from build123d import *

# Parameters (mm, degrees)
SKETCH_1_R               = 1.1
EXTRUDE_2_DEPTH          = 4.5
FILLET_1_R               = 7
FILLET_2_R               = 14
FILLET_3_R               = 2
CUT_EXTRUDE_1_DEPTH      = 33.524221985
CUT_EXTRUDE_1_DEPTH_BACK = 33.524221985


with BuildPart() as part:
    # 草图1 → 凸台-拉伸2 (new body)
    with BuildSketch(Plane.XY):
        with BuildLine():
            Line((6.017486991, 19.788810031), (-7.057549395, 16.285364591))
            Line((-7.057549395, 16.285364591), (-7.057549395, -16.139577348))
            Line((-7.057549395, -16.139577348), (-7.057549395, -28.167744528))
            Line((-7.057549395, -28.167744528), (6.017486991, -31.671189969))
            Line((6.017486991, -31.671189969), (7.089384541, -30.477023749))
            ThreePointArc((7.089384541, -30.477023749), (3.917486991, -28.671189969), (7.089384541, -26.865356188))
            Line((7.089384541, -26.865356188), (6.017486991, -25.671189969))
            Line((6.017486991, -25.671189969), (-2.887475269, -24.892106722))
            Line((-2.887475269, -24.892106722), (-2.887475269, 13.009726784))
            Line((-2.887475269, 13.009726784), (6.017486991, 13.788810031))
            Line((6.017486991, 13.788810031), (7.089384541, 14.982976251))
            ThreePointArc((7.089384541, 14.982976251), (3.917486991, 16.788810031), (7.089384541, 18.594643812))
            Line((7.089384541, 18.594643812), (6.017486991, 19.788810031))
        make_face()
        with Locations((-4.879152463, 4.788810031)):
            Circle(SKETCH_1_R, mode=Mode.SUBTRACT)
        with Locations((-4.879152463, -16.671189969)):
            Circle(SKETCH_1_R, mode=Mode.SUBTRACT)
    extrude(amount=EXTRUDE_2_DEPTH)

    # 圆角1
    fillet_1_edges = [part.edges().sort_by_distance(p)[0] for p in [
        (-2.887475269, 13.009726784, 2.25),
        (-2.887475269, -24.892106722, 2.25),
    ]]
    fillet(fillet_1_edges, radius=FILLET_1_R)

    # 圆角2
    fillet_2_edges = [part.edges().sort_by_distance(p)[0] for p in [
        (-7.057549395, -28.167744528, 2.25),
        (-7.057549395, 16.285364591, 2.25),
    ]]
    fillet(fillet_2_edges, radius=FILLET_2_R)

    # 圆角3
    fillet_3_edges = [part.edges().sort_by_distance(p)[0] for p in [
        (6.017486991, 13.788810031, 2.25),
        (6.017486991, -25.671189969, 2.25),
        (6.017486991, -31.671189969, 2.25),
        (6.017486991, 19.788810031, 2.25),
    ]]
    fillet(fillet_3_edges, radius=FILLET_3_R)

    # 草图2 → 切除-拉伸1 (cut, two sides: drawn at the far end of the back side and taken through both)
    with BuildSketch(Plane(origin=(0, 0, 0), x_dir=(1, 0, 0), z_dir=(0, 1, 0)).offset(-CUT_EXTRUDE_1_DEPTH_BACK)):
        Polygon((-9.937735325, -0.89235354), (-9.653427695, 2.8886559), (6.091848462, 2.8886559), (7.089384541, 0), (-4.928773799, -0.62984499), (-9.504604651, -0.62984499), align=None)
        Polygon((7.089384541, -4.5), (-9.927872999, -3.608163323), (-9.667318366, -5.613598375), (7.089384541, -5.407507841), align=None)
    extrude(amount=CUT_EXTRUDE_1_DEPTH + CUT_EXTRUDE_1_DEPTH_BACK, mode=Mode.SUBTRACT)


solid = part.part
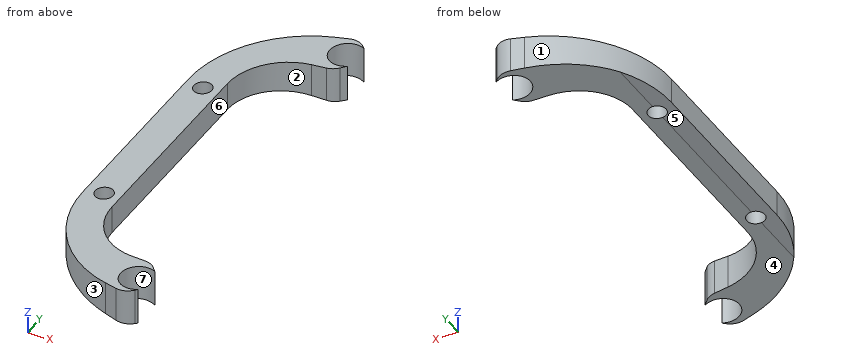
Model file for the job. Use its own axes, mm. Face numbers are marked on the shaded views. A direction names the side the tool comes from. Round coordinates to 2 decimals unless told otherwise and drop trailing zeros. Order: outer loops, then holes, each group sorted by start corner. A loop starts at its lowest first (then second) coordinate and runs counter-clockwise, first axis right, second up. Notation, with made-up numbers: M 25,56.5 L 40,56.5 A5 cw 40,60.5 Z; hole C 6.5,47.25 d8. An arc over 180 degrees is marked long. Write each question's results on one line, items separated by ' | '. Start each with the question number.
(1) Saw through at A-A, the plane x = -1. Give the cut face in (y, z), then the cut area to 3 significant figures.
(2) Two-plate mould, pull along Y, no slides. Class the marked faces 1, 2, 3 and 4: pulls with the +Y half, pulls with the -Y half, needs draft (parallel to the pull), parting line crosses it, or undercut.
(3) Saw through at B-B, the plane x = 6. Give the cut face in (y, z).
(4) Saw through at D-D, the plane y = -5. Give the cut face in (x, z).
(5) Drop flat-ended pins along their axis: pin 1 (3 mm diameter, centred on x = -4.88, y = 4.79, fed in from +Z); pin 2 (1 mm diameter, centred on y = -6, z = 3, fed in from +X); pin 3 (0.6 mm diameter, centred on x = -6, y = -2.5, fed in from -Z). Give the stop position or say it passes through.
(6) Saw through at C-C, the plane z = 2.95. Give the cut face in (x, y).
(7) Which spindle directions (+Z, -Z, +X, -X, +Y, -Y) get a long thin tool onto all of the face, cutting with end or side? Do the marked faces 5, 6 and 7. Say none if no direction does.
(8) Probe probe 1 along Y at (x, z) = (-5, 3.6); probe 2 along Y at (x, z) = (-5.5, 1.9); probe 3 along X at (y, z) = (-5, 2.65). List the from-to ranges inside material, lowest first. Write a range as from..to.
Established:
1) outline: M -28.95,0.42 L -23.26,0.42 L -23.26,4.08 L -28.95,4.08 Z; M 11.38,0.42 L 17.07,0.42 L 17.07,4.08 L 11.38,4.08 Z | area: 41.6 mm^2
2) face 1: pulls with the +Y half | face 2: undercut | face 3: pulls with the -Y half | face 4: needs draft
3) outline: M -31.31,0.06 L -30.77,0.06 L -30.77,4.44 L -31.31,4.44 Z; M -26.57,0.06 L -25.83,0.06 L -25.83,4.44 L -26.57,4.44 Z; M 13.95,0.06 L 14.69,0.06 L 14.69,4.44 L 13.95,4.44 Z; M 18.89,0.06 L 19.43,0.06 L 19.43,4.44 L 18.89,4.44 Z
4) outline: M -7.06,0.63 L -4.93,0.63 L -2.89,0.52 L -2.89,3.98 L -7.06,3.76 Z
5) pin 1: stops at z = 3.95 | pin 2: stops at x = -2.89 | pin 3: stops at z = 0.63
6) outline: M -7.06,-17.43 A14 ccw 3.32,-30.95 L 4.83,-31.35 A2 ccw 6.84,-30.76 L 7.09,-30.48 A2.1 cw long 7.09,-26.87 L 6.54,-26.26 A2 ccw 5.23,-25.6 L 3.5,-25.45 A7 cw -2.89,-18.48 L -2.89,6.6 A7 cw 3.5,13.57 L 5.23,13.72 A2 ccw 6.54,14.38 L 7.09,14.98 A2.1 cw long 7.09,18.59 L 6.84,18.88 A2 ccw 4.83,19.47 L 3.32,19.07 A14 ccw -7.06,5.54 Z; hole C -4.88,-16.67 d2.2; hole C -4.88,4.79 d2.2
7) face 5: -Z, -X, +Y, -Y | face 6: +Z, -Z, +X | face 7: +Z, -Z
8) probe 1: y = -24.73..-17.76, -15.58..3.7, 5.88..12.85 | probe 2: y = -23.84..-17.58, -15.76..3.88, 5.7..11.96 | probe 3: x = -7.06..-2.89
